```python
from build123d import *

# Parameters (mm, degrees)
F1_DEPTH  = 31.75
F2_R      = 6.35
F3_W      = 13.97
F3_H      = 25.4
F4_DEPTH  = 12.7
F5_R      = 3.175
F6_DEPTH  = 8.891
F7_R      = 3.175
F8_DEPTH  = 8.891
F10_DEPTH = 1.27


with BuildPart() as f1:
    # F0 (on Right) → F1 (new body)
    with BuildSketch(Plane.YZ):
        with BuildLine():
            Line((5.08, 22.86), (-5.08, 22.86))
            ThreePointArc((-5.08, 22.86), (-37.4089220358, 9.4689220358), (-50.8, -22.86))
            Line((-50.8, -22.86), (-49.3431158517, -22.86))
            Line((-49.3431158517, -22.86), (-48.3434804291, -22.86))
            ThreePointArc((-48.3434804291, -22.86), (-35.2079259795, -19.1997610222), (-25.8581406946, -9.2739534884))
            ThreePointArc((-25.8581406946, -9.2739534884), (2.5656373666, 6.2371064696), (27.8365726971, -14.0084848485))
            ThreePointArc((27.8365726971, -14.0084848485), (32.4422895224, -20.410994039), (39.9394303915, -22.86))
            Line((39.9394303915, -22.86), (50.8, -22.86))
            ThreePointArc((50.8, -22.86), (37.4089220358, 9.4689220358), (5.08, 22.86))
        make_face()
        Polygon((-49.3431158517, -22.86), (-50.8, -22.86), (-50.0715579258, -23.9003230962), align=None)
    extrude(amount=F1_DEPTH)

    # F2
    f2_edges = [f1.edges().sort_by_distance(p)[0] for p in [
        (15.875, 50.8, -22.86),
    ]]
    fillet(f2_edges, radius=F2_R)

    # F3 (on face) → F4 (cut)
    with BuildSketch(Plane(origin=(0, 0, -22.86), x_dir=(1, 0, 0), z_dir=(0, 0, -1))):
        with Locations((15.875, -41.9369795426)):
            Rectangle(F3_W, F3_H)
    extrude(amount=-F4_DEPTH, mode=Mode.SUBTRACT)

    # F5 (on face) → F6 (cut, through all)
    with BuildSketch(Plane.YZ.offset(8.89)):
        with Locations((43.9345286936, -16.51)):
            Circle(F5_R)
    extrude(amount=-F6_DEPTH, mode=Mode.SUBTRACT)

    # F7 (on face) → F8 (cut, through all)
    with BuildSketch(Plane(origin=(22.86, 0, 0), x_dir=(0, -1, 0), z_dir=(-1, 0, 0))):
        with Locations((-43.9345286936, -16.51)):
            Circle(F7_R)
    extrude(amount=-F8_DEPTH, mode=Mode.SUBTRACT)

    # F9 (on face) → F10 (cut)
    with BuildSketch(Plane(origin=(0, -44.8279982961, -31.3889023298), x_dir=(1, 0, 0), z_dir=(0, -0.8191520443, -0.5735764364))):
        Polygon((0.5291666667, 10.4118672342), (0, 9.1418672342), (1.0583333333, 9.1418672342), align=None)
        Polygon((31.2208333333, 10.4118672342), (30.6916666667, 9.1418672342), (31.75, 9.1418672342), align=None)
        Polygon((30.1625, 10.4118672342), (29.6333333333, 9.1418672342), (30.6916666667, 9.1418672342), align=None)
        Polygon((29.1041666667, 10.4118672342), (28.575, 9.1418672342), (29.6333333333, 9.1418672342), align=None)
        Polygon((28.0458333333, 10.4118672342), (27.5166666667, 9.1418672342), (28.575, 9.1418672342), align=None)
        Polygon((26.9875, 10.4118672342), (26.4583333333, 9.1418672342), (27.5166666667, 9.1418672342), align=None)
        Polygon((25.9291666667, 10.4118672342), (25.4, 9.1418672342), (26.4583333333, 9.1418672342), align=None)
        Polygon((24.8708333333, 10.4118672342), (24.3416666667, 9.1418672342), (25.4, 9.1418672342), align=None)
        Polygon((23.8125, 10.4118672342), (23.2833333333, 9.1418672342), (24.3416666667, 9.1418672342), align=None)
        Polygon((22.7541666667, 10.4118672342), (22.225, 9.1418672342), (23.2833333333, 9.1418672342), align=None)
        Polygon((21.6958333333, 10.4118672342), (21.1666666667, 9.1418672342), (22.225, 9.1418672342), align=None)
        Polygon((20.6375, 10.4118672342), (20.1083333333, 9.1418672342), (21.1666666667, 9.1418672342), align=None)
        Polygon((19.5791666667, 10.4118672342), (19.05, 9.1418672342), (20.1083333333, 9.1418672342), align=None)
        Polygon((18.5208333333, 10.4118672342), (17.9916666667, 9.1418672342), (19.05, 9.1418672342), align=None)
        Polygon((17.4625, 10.4118672342), (16.9333333333, 9.1418672342), (17.9916666667, 9.1418672342), align=None)
        Polygon((16.4041666667, 10.4118672342), (15.875, 9.1418672342), (16.9333333333, 9.1418672342), align=None)
        Polygon((15.3458333333, 10.4118672342), (14.8166666667, 9.1418672342), (15.875, 9.1418672342), align=None)
        Polygon((14.2875, 10.4118672342), (13.7583333333, 9.1418672342), (14.8166666667, 9.1418672342), align=None)
        Polygon((13.2291666667, 10.4118672342), (12.7, 9.1418672342), (13.7583333333, 9.1418672342), align=None)
        Polygon((12.1708333333, 10.4118672342), (11.6416666667, 9.1418672342), (12.7, 9.1418672342), align=None)
        Polygon((11.1125, 10.4118672342), (10.5833333333, 9.1418672342), (11.6416666667, 9.1418672342), align=None)
        Polygon((10.0541666667, 10.4118672342), (9.525, 9.1418672342), (10.5833333333, 9.1418672342), align=None)
        Polygon((8.9958333333, 10.4118672342), (8.4666666667, 9.1418672342), (9.525, 9.1418672342), align=None)
        Polygon((7.9375, 10.4118672342), (7.4083333333, 9.1418672342), (8.4666666667, 9.1418672342), align=None)
        Polygon((6.8791666667, 10.4118672342), (6.35, 9.1418672342), (7.4083333333, 9.1418672342), align=None)
        Polygon((5.8208333333, 10.4118672342), (5.2916666667, 9.1418672342), (6.35, 9.1418672342), align=None)
        Polygon((4.7625, 10.4118672342), (4.2333333333, 9.1418672342), (5.2916666667, 9.1418672342), align=None)
        Polygon((3.7041666667, 10.4118672342), (3.175, 9.1418672342), (4.2333333333, 9.1418672342), align=None)
        Polygon((2.6458333333, 10.4118672342), (2.1166666667, 9.1418672342), (3.175, 9.1418672342), align=None)
        Polygon((1.5875, 10.4118672342), (1.0583333333, 9.1418672342), (2.1166666667, 9.1418672342), align=None)
    extrude(amount=-F10_DEPTH, mode=Mode.SUBTRACT)


solid = f1.part
```
Geometry check sheet. Reference: the model listing, model coordinates, mm. A direction names the side the tool comes from. Give positions to 0.01 mm unless a question says otherwise; leave off trailing zeros. Loops run counter-clockwise (first coordinate to the right, second up) from the corner with the lowest first, then second, coordinate; pieces in that order, holes last. Notation, with made-up numbers: (51.25, 73.25) - (107.25, 73.25) arc R10 cw to (107.25, 91.25) - close; hole circle Ø8 at (-13.5, 10). An arc over 180 degrees is marked (long way). Use CSV: the item, a comma, the result in double quotes. Start each with the question number.
Q1. Go/stop test with flat-tipped pins: pin 1 Ø4 at (x, z) = (28.5, -6.5) entering from +Y; pin 2 Ø8 at (x, y) = (10, 37) entering from +Z; pin 3 Ø1.5 at (x, y) = (14, 29.5) entering from -Z; pin 4 Ø4 at (y, z) = (43.93, -16.51) entering from -X. Record where each tip stops, or that it passes through.
Q2. Section check D-D, the plane y = 8. Record the cut outline in (x, z), and give its area (3 significant figures).
Q3. Section check C-C, the plane z = 14. Record the cut outline in (x, y), and give its area (3 significant figures).
Q4. Section check B-B, the plane y = 32.5. Record the cut outline in (x, z) (3 decimals), and give its area (3 significant figures).
Q5. Access from +Z, -Z, +X, -X, +Y, -Y to the whole of each face (thin tool, end or side, straight path). Record for faces 1 (the face through (16, 39, -10.16)), 2 (the face through (4, 42, -22.86)), 3 (the face through (15.65, 28.85, -16.35)).
Q6. Scan lines: probe 1 along Z at (x, y) = (25, 42); probe 2 along Z at (x, y) = (23, 0); probe 3 along Y at (x, z) = (24, -5). Record each from-to range of solid material in increasing order. Write a range as from..to.
Q7. Release check for a two-part mould opening along Y. For faces 4 (the face through (15.653, -35.374, -19.299)), 5 (the face through (27.243, 41.002, -17.726)), 6 (the face through (4.507, 48.723, -20.68)), 7 (the face through (8.89, 40, -17)) record: +Y half, -Y half, draft (parallel to the pull), parting line (faces both ways), or undercut.
Q8. Section check A-A, the plane z = -4. Record the cut outline in (x, y), and give its area (3 significant figures).
Findings below:
1,pin 1,"stops at y = 48.49"
1,pin 2,"stops at z = 13.34"
1,pin 3,"stops at z = -17"
1,pin 4,"passes through"
2,outline,"(0, 5.23) - (31.75, 5.23) - (31.75, 22.77) - (0, 22.77) - close"
2,area,"557 mm^2"
3,outline,"(0, -32.13) - (31.75, -32.13) - (31.75, 32.13) - (0, 32.13) - close"
3,area,"2,040 mm^2"
4,outline,"(0, -20.453) - (8.89, -20.453) - (8.89, -10.16) - (22.86, -10.16) - (22.86, -20.453) - (31.75, -20.453) - (31.75, 13.725) - (0, 13.725) - close"
4,area,"941 mm^2"
5,face 1,"-Z, +Y"
5,face 2,"-Z, +X, -X, +Y"
5,face 3,"-Z, +X, -X"
6,probe 1,"z = -22.86..-19.03, -13.99..4.11"
6,probe 2,"z = 6.35..22.86"
6,probe 3,"y = -47.17..-23.11, 23.11..47.17"
7,face 4,"undercut"
7,face 5,"undercut"
7,face 6,"+Y half"
7,face 7,"draft"
8,outline,"(0, -46.73) - (31.75, -46.73) - (31.75, -22.31) - (0, -22.31) - close; (0, 22.31) - (31.75, 22.31) - (31.75, 46.73) - (0, 46.73) - close"
8,area,"1,550 mm^2"
